Autodesk Inventor part; units mm, degrees
ref_plane "YZ Plane" through (0, 0, 0) normal (1, 0, 0) x (0, 1, 0)
ref_plane "XZ Plane" through (0, 0, 0) normal (0, 1, 0) x (-1, 0, 0)
ref_plane "XY Plane" through (0, 0, 0) normal (0, 0, 1) x (1, 0, 0)
sketch "スケッチ1" plane through (0, 0, 0) normal (0, 0, 1) x (1, 0, 0)
  line L0 (-40, -55) -> (40, -55)
  line L1 (40, -55) -> (40, 55)
  line L2 (40, 55) -> (-40, 55)
  line L3 (-40, 55) -> (-40, -55)
  line L4 (-40, -55) -> (40, 55) construction
  line L5 (40, -55) -> (-40, 55) construction
  circle A0 centre (10, 43) radius 4.6
  circle A1 centre (25, 25) radius 5
  circle A2 centre (25, 25) radius 12.5 construction
  circle A3 centre (10, 43) radius 8.25 construction
  line L6 (0, -77) -> (0, 77) construction
  circle A4 centre (0, -15) radius 32.75 construction
  line L7 (-36, 20) -> (4, 20) construction
  line L8 (4, 20) -> (4, 36) construction
  line L9 (4, 36) -> (-36, 36) construction
  line L10 (-36, 36) -> (-36, 20) construction
  line L11 (-36, 20) -> (4, 36) construction
  line L12 (4, 20) -> (-36, 36) construction
  line L13 (13.4369, 50.5) -> (21.75, 50.5) construction
  line L14 (21.75, 50.5) -> (21.75, 35.5) construction
  line L15 (21.75, 35.5) -> (13.4369, 35.5) construction
  line L16 (8.5, 32.5) -> (8.5, 35)
  line L17 (8.5, 35) -> (11.5, 35)
  line L18 (11.5, 35) -> (11.5, 32.5)
  line L19 (8.5, 32.5) -> (11.5, 32.5)
  line L20 (8.5, 35) -> (11.5, 32.5) construction
  line L21 (11.5, 35) -> (8.5, 32.5) construction
  line L22 (0, -15) -> (28.3623, 1.375) construction
  line L23 (0, -15) -> (-28.3623, 1.375) construction
  circle A5 centre (0, -15) radius 36 construction
  circle A6 centre (31.1769, 3) radius 1.6
  circle A7 centre (-31.1769, 3) radius 1.6
  circle A8 centre (0, -51) radius 1.6
  line L24 (-32.75, -15) -> (32.75, -15) construction
  circle A9 centre (-4, -15) radius 2.5
  circle A10 centre (0, -8.0718) radius 2.5
  circle A11 centre (4, -15) radius 2.5
  circle A12 centre (8, -8.0718) radius 2.5
  circle A13 centre (-12, -15) radius 2.5
  circle A14 centre (-8, -8.0718) radius 2.5
  circle A15 centre (12, -15) radius 2.5
  circle A16 centre (16, -8.0718) radius 2.5
  circle A17 centre (-20, -15) radius 2.5
  circle A18 centre (-16, -8.0718) radius 2.5
  circle A19 centre (20, -15) radius 2.5
  circle A20 centre (24, -8.0718) radius 2.5
  circle A21 centre (-4, -1.1436) radius 2.5
  circle A22 centre (0, 5.7846) radius 2.5
  circle A23 centre (4, -1.1436) radius 2.5
  circle A24 centre (8, 5.7846) radius 2.5
  circle A25 centre (-12, -1.1436) radius 2.5
  circle A26 centre (-8, 5.7846) radius 2.5
  circle A27 centre (12, -1.1436) radius 2.5
  circle A28 centre (16, 5.7846) radius 2.5
  circle A29 centre (-20, -1.1436) radius 2.5
  circle A30 centre (-16, 5.7846) radius 2.5
  circle A31 centre (20, -1.1436) radius 2.5
  circle A32 centre (24, 5.7846) radius 2.5 construction
  circle A33 centre (-4, -28.8564) radius 2.5
  circle A34 centre (0, -21.9282) radius 2.5
  circle A35 centre (4, -28.8564) radius 2.5
  circle A36 centre (8, -21.9282) radius 2.5
  circle A37 centre (-12, -28.8564) radius 2.5
  circle A38 centre (-8, -21.9282) radius 2.5
  circle A39 centre (12, -28.8564) radius 2.5
  circle A40 centre (16, -21.9282) radius 2.5
  circle A41 centre (-20, -28.8564) radius 2.5
  circle A42 centre (-16, -21.9282) radius 2.5
  circle A43 centre (20, -28.8564) radius 2.5
  circle A44 centre (24, -21.9282) radius 2.5
  circle A45 centre (-4, 12.7128) radius 2.5
  circle A46 centre (0, 19.641) radius 2.5 construction
  circle A47 centre (4, 12.7128) radius 2.5
  circle A48 centre (8, 19.641) radius 2.5 construction
  circle A49 centre (-12, 12.7128) radius 2.5 construction
  circle A50 centre (-8, 19.641) radius 2.5 construction
  circle A51 centre (12, 12.7128) radius 2.5 construction
  circle A52 centre (16, 19.641) radius 2.5 construction
  circle A53 centre (-20, 12.7128) radius 2.5 construction
  circle A54 centre (-16, 19.641) radius 2.5 construction
  circle A55 centre (20, 12.7128) radius 2.5 construction
  circle A56 centre (24, 19.641) radius 2.5 construction
  circle A57 centre (-4, -42.7128) radius 2.5
  circle A58 centre (0, -35.7846) radius 2.5
  circle A59 centre (4, -42.7128) radius 2.5
  circle A60 centre (8, -35.7846) radius 2.5
  circle A61 centre (-12, -42.7128) radius 2.5 construction
  circle A62 centre (-8, -35.7846) radius 2.5
  circle A63 centre (12, -42.7128) radius 2.5 construction
  circle A64 centre (16, -35.7846) radius 2.5
  circle A65 centre (-20, -42.7128) radius 2.5 construction
  circle A66 centre (-16, -35.7846) radius 2.5
  circle A67 centre (20, -42.7128) radius 2.5 construction
  circle A68 centre (24, -35.7846) radius 2.5 construction
  circle A69 centre (0, -15) radius 30 construction
  circle A70 centre (-28, -15) radius 2.5
  circle A71 centre (-24, -8.0718) radius 2.5
  circle A72 centre (-28, -1.1436) radius 2.5 construction
  circle A73 centre (-24, 5.7846) radius 2.5 construction
  circle A74 centre (-28, -28.8564) radius 2.5 construction
  circle A75 centre (-24, -21.9282) radius 2.5
  circle A76 centre (-28, 12.7128) radius 2.5 construction
  circle A77 centre (-24, 19.641) radius 2.5 construction
  circle A78 centre (-28, -42.7128) radius 2.5 construction
  circle A79 centre (-24, -35.7846) radius 2.5 construction
  circle A80 centre (28, -15) radius 2.5
  circle A81 centre (32, -8.0718) radius 2.5 construction
  circle A82 centre (28, -1.1436) radius 2.5 construction
  circle A83 centre (32, 5.7846) radius 2.5 construction
  circle A84 centre (28, -28.8564) radius 2.5 construction
  circle A85 centre (32, -21.9282) radius 2.5 construction
  circle A86 centre (28, 12.7128) radius 2.5 construction
  circle A87 centre (32, 19.641) radius 2.5 construction
  circle A88 centre (28, -42.7128) radius 2.5 construction
  circle A89 centre (32, -35.7846) radius 2.5 construction
  circle A90 centre (-33, 33) radius 1.35
  circle A91 centre (1, 33) radius 1.35
  point P0 (0, 0)
  point P1 (-16, 28)
  point P2 (10, 33.75)
  point P3 (10, 33.75)
  dimension "d32" = 72
  dimension "d0" = 110
  dimension "d1" = 80
  dimension "d2" = 12
  dimension "d3" = 9.2
  dimension "d5" = 30
  dimension "d6" = 15
  dimension "d7" = 30
  dimension "d8" = 25
  dimension "d9" = 10
  dimension "d10" = 25
  dimension "d11" = 16.5
  dimension "d12" = 65.5
  dimension "d15" = 15
  dimension "d16" = 40
  dimension "d17" = 16
  dimension "d19" = 4
  dimension "d20" = 35
  dimension "d21" = 40
  dimension "d22" = 58
  dimension "d23" = 15
  dimension "d24" = 11.75
  dimension "d27" = 3
  dimension "d29" = 8
  dimension "d30" = 2.5
  dimension "d31" = 120
  dimension "d33" = 3.2
  dimension "d36" = 360
  dimension "d38" = 5
  dimension "d39" = 8
  dimension "d43" = 8
  dimension "d46" = 13.8564
  dimension "d49" = 8
  dimension "d50" = 60
  dimension "d51" = 2.7
  dimension "d52" = 3
  dimension "d53" = 3
  dimension "d54" = 3
  dimension "d55" = 3
  dimension "d61" = 10
extrude "押し出し1" add sketch "スケッチ1" along normal blind 4
chamfer "面取り1" distance 2 angle 45 4 edges at (40, 55, 2) (-40, 55, 2) (-40, -55, 2) (40, -55, 2)
sketch "スケッチ2" plane through (0, 0, 4) normal (0, 0, 1) x (1, 0, 0)
  line L0 (36, -51) -> (-36, -51) construction
  line L1 (-36, -51) -> (-36, 51) construction
  line L2 (-36, 51) -> (36, 51) construction
  line L3 (36, 51) -> (36, -51) construction
  line L4 (36, -51) -> (-36, 51) construction
  line L5 (-36, -51) -> (36, 51) construction
  circle A0 centre (-36, 51) radius 1.6
  circle A1 centre (36, 51) radius 1.6
  circle A2 centre (-36, -51) radius 1.6
  circle A3 centre (36, -51) radius 1.6
  line L6 (-40, 53) -> (-40, -53) construction
  line L7 (38, 55) -> (-38, 55) construction
  point P0 (0, 0)
  dimension "d62" = 3.2
  dimension "d63" = 4
  dimension "d64" = 4
extrude "押し出し2" cut sketch "スケッチ2" against normal through all
equation "\"d39\" = d43"
equation "\"d49\" = d43"
equation "\"d64\" = d63"
properties part number "front_pannel" material "PMMA プラスチック"
Geometry check sheet. Reference: the model listing, model coordinates, mm. Give positions to 0.01 mm unless a question says otherwise; leave off trailing zeros. Write each loop counter-clockwise with the first axis right and the second up, starting at its lowest first coordinate (ties: lowest second). Pieces come first, ordered by that corner, then holes.
1) Cross-section at A-A (x = -12). Record the boundary of the cut face in (y, z), plus the area to 3 significant figures.
Values follow:
outline: (-55, 0) - (-31.36, 0) - (-31.36, 4) - (-55, 4) - close; (-26.36, 0) - (-17.5, 0) - (-17.5, 4) - (-26.36, 4) - close; (-12.5, 0) - (-3.64, 0) - (-3.64, 4) - (-12.5, 4) - close; (1.36, 0) - (55, 0) - (55, 4) - (1.36, 4) - close
area: 380 mm2
2) Thickness scan on line 1 (X direction, y = 6, z = 2.45); line 2 (Y direction, x = 16, z = 2.5); line 3 (Y direction, x = -12, z = 1.85). Record the ranges inside material, lowest first.
Values follow:
line 1: x = -40 to -18.49, -13.51 to -10.49, -5.51 to -2.49, 2.49 to 5.51, 10.49 to 13.51, 18.49 to 40
line 2: y = -55 to -38.28, -33.28 to -24.43, -19.43 to -10.57, -5.57 to 3.28, 8.28 to 55
line 3: y = -55 to -31.36, -26.36 to -17.5, -12.5 to -3.64, 1.36 to 55
3) Cross-section at D-D (x = 16). Record the boundary of the cut face in (y, z), plus the area to 3 significant figures.
Values follow:
outline: (-55, 0) - (-38.28, 0) - (-38.28, 4) - (-55, 4) - close; (-33.28, 0) - (-24.43, 0) - (-24.43, 4) - (-33.28, 4) - close; (-19.43, 0) - (-10.57, 0) - (-10.57, 4) - (-19.43, 4) - close; (-5.57, 0) - (3.28, 0) - (3.28, 4) - (-5.57, 4) - close; (8.28, 0) - (55, 0) - (55, 4) - (8.28, 4) - close
area: 360 mm2
4) Cross-section at C-C (y = -51). Record the boundary of the cut face in (x, z), plus the area to 3 significant figures.
Values follow:
outline: (-40, 0) - (-37.6, 0) - (-37.6, 4) - (-40, 4) - close; (-34.4, 0) - (-1.6, 0) - (-1.6, 4) - (-34.4, 4) - close; (1.6, 0) - (34.4, 0) - (34.4, 4) - (1.6, 4) - close; (37.6, 0) - (40, 0) - (40, 4) - (37.6, 4) - close
area: 282 mm2
5) Release check for a two-part mould opening along Y. For faces 1 (the face through (-1, -55, 2)), 2 (the face through (-22.5, -15.1, 2)), 3 (the face through (9.5, -15.1, 2)) record: released by +Y, released by -Y, zero draft, split by the parting line, or undercut.
Values follow:
face 1: released by -Y
face 2: undercut
face 3: undercut
6) Cross-section at B-B (x = -24). Record the boundary of the cut face in (y, z), plus the area to 3 significant figures.
Values follow:
outline: (-55, 0) - (-24.43, 0) - (-24.43, 4) - (-55, 4) - close; (-19.43, 0) - (-10.57, 0) - (-10.57, 4) - (-19.43, 4) - close; (-5.57, 0) - (55, 0) - (55, 4) - (-5.57, 4) - close
area: 400 mm2
